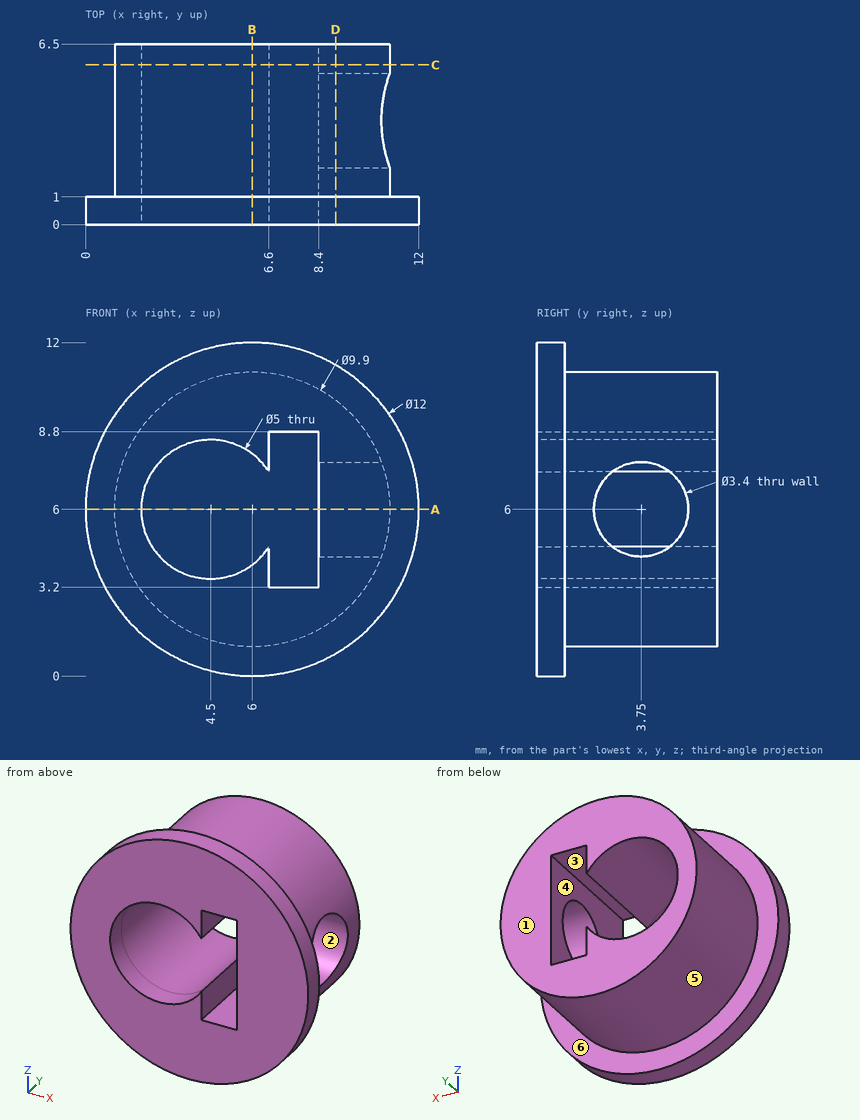
Check sheet for the drawn part. Datum: minimum x, y, z corner. Units: mm. A direction names the side the tool comes from. Round coordinates to 2 decimals unless told otherwise and drop trailing zeros. Loops run counter-clockwise (first coordinate to the right, second up) from the corner with the lowest first, then second, coordinate; pieces in that order, holes last. Notation, with made-up numbers: M 42,49.25 L 60,49.25 A14 ccw 60,56.25 Z; hole C 69,-35 d6. An arc over 180 degrees is marked long. Write each question's results on one line, items separated by ' | '.
1) Gauge pin test, flat ends, axial feed: P1, Ø2, axis at y = 1, z = 4, coming from the +X side; P2, Ø3, axis at x = 7.5, y = 4.5, coming from the +Z side; P3, Ø2, axis at x = 10, y = 3, coming from the +Z side. Record the tip position at first contact, or that the pin passes through.
Checks:
P1: stops at x = 11.92 | P2: stops at z = 10.95 | P3: stops at z = 9.94
2) Section check D-D on x = 9. Record the boundary of the cut face in (y, z).
Checks:
outline: M 0,0.8 L 1,0.8 L 1,2.06 L 6.5,2.06 L 6.5,9.94 L 1,9.94 L 1,11.2 L 0,11.2 Z; hole C 3.75,6 d3.4
3) Section check C-C on y = 5.75. Record the boundary of the cut face in (x, z).
Checks:
outline: C 6,6 d9.9; hole M 6.6,3.2 L 8.4,3.2 L 8.4,8.8 L 6.6,8.8 L 6.6,7.36 A2.5 ccw long 6.6,4.64 Z
4) Section check B-B on x = 6. Record the boundary of the cut face in (y, z).
Checks:
outline: M 0,0 L 1,0 L 1,1.05 L 6.5,1.05 L 6.5,4 L 0,4 Z; M 0,8 L 6.5,8 L 6.5,10.95 L 1,10.95 L 1,12 L 0,12 Z
5) Section check A-A on z = 6. Record the boundary of the cut face in (x, y), then the cut area to 3 significant figures.
Checks:
outline: M 0,0 L 2,0 L 2,6.5 L 1.05,6.5 L 1.05,1 L 0,1 Z; M 8.4,0 L 12,0 L 12,1 L 10.95,1 L 10.95,2.05 L 8.4,2.05 Z; M 8.4,5.45 L 10.95,5.45 L 10.95,6.5 L 8.4,6.5 Z | area: 16.2 mm2
6) Access from +Z, -Z, +X, -X, +Y, -Y to the whole of each face (thin tool, end or side, straight path). Record for the marked faces 1, 2 and 3.
Checks:
face 1: +Z, -Z, +X, -X, +Y | face 2: +X | face 3: +Y, -Y
7) Scan lines: L1, parallel to Y at x = 9.4, z = 6; L2, parallel to Y at x = 1, z = 3.25; L3, parallel to X at y = 0.5, z = 6. Record each from-to range of solid material in increasing order. Write a range as from..to.
Checks:
L1: y = 0..2.05, 5.45..6.5 | L2: y = 0..1 | L3: x = 0..2, 8.4..12
8) Mould release check, pull along X, two halves, no side actions. Record for the marked faces 4, 5 and 6: released by +X, released by -X, zero draft, split by the parting line, or undercut.
Checks:
face 4: undercut | face 5: split by the parting line | face 6: zero draft
